Build history of the part. All positions in model axes, mm. Coordinates: 2 decimals unless noted, no trailing zeros. Loops run counter-clockwise (first coordinate to the right, second up) from the corner with the lowest first, then second, coordinate; pieces in that order, holes last.
Item 1: Cut at D-D (x = 8.5). List the corners of the cut face in (y, z).
Item 2: Cut at B-B (x = -11). List the corners of the cut face in (y, z), and give its area (3 significant figures).
Item 3: Drill centre lines: line 1 along Y through (x, z) = (-11, 1); line 2 along X through (y, z) = (-13, 1); line 3 along X through (y, z) = (-10, 1.25). Where is each one in solid material? Low to high.
Item 4: Cut at A-A (y = -13). List the corners of the cut face in (x, z).
Item 5: Cut at C-C (z = 2.3). List the corners of the cut face in (x, y), and give its area (3 significant figures).
Item 6: Mould opens along Y. For faces 1 (the face through (0, 0, 0)), 2 (the face through (-12.5, 13.07, 1.52)), 3 (the face through (0, -20, 1)), 4 (the face through (9.526, -11.352, 1.521)) say: released by +Y, released by -Y, zero draft, split by the parting line, or undercut.
from build123d import *

# Parameters (mm, degrees)
ESQUISSE1_W             = 28
ESQUISSE1_H             = 40
BOSS_EXTRU_1_DEPTH      = 3
ESQUISSE7_R             = 1.5
ENL_V_MAT_EXTRU_6_DEPTH = 5
ESQUISSE8_R             = 2
ENL_V_MAT_EXTRU_7_DEPTH = 10
ESQUISSE9_R             = 6
ENL_V_MAT_EXTRU_8_DEPTH = 10


with BuildPart() as part:
    # Esquisse1 → Boss.-Extru.1 (new body)
    with BuildSketch(Plane.XY):
        Rectangle(ESQUISSE1_W, ESQUISSE1_H)
    extrude(amount=BOSS_EXTRU_1_DEPTH)

    # Esquisse7 → Enlèv. mat.-Extru.6 (cut)
    with BuildSketch(Plane.XY.offset(3)):
        with Locations((-11, 13)):
            Circle(ESQUISSE7_R)
    enl_v_mat_extru_6 = extrude(amount=-ENL_V_MAT_EXTRU_6_DEPTH, mode=Mode.SUBTRACT)

    # Symétrie2: Enlèv. mat.-Extru.6 across plane
    add(enl_v_mat_extru_6.mirror(Plane.ZX), mode=Mode.SUBTRACT)

    # Esquisse8 → Enlèv. mat.-Extru.7 (cut)
    with BuildSketch(Plane.XY.offset(3)):
        with Locations((11, 10)):
            Circle(ESQUISSE8_R)
    enl_v_mat_extru_7 = extrude(amount=-ENL_V_MAT_EXTRU_7_DEPTH, mode=Mode.SUBTRACT)

    # Symétrie3: Enlèv. mat.-Extru.7 across plane
    add(enl_v_mat_extru_7.mirror(Plane.ZX), mode=Mode.SUBTRACT)

    # Esquisse9 → Enlèv. mat.-Extru.8 (cut)
    with BuildSketch(Plane.XY.offset(3)):
        with Locations((14, 0)):
            Circle(ESQUISSE9_R)
    extrude(amount=-ENL_V_MAT_EXTRU_8_DEPTH, mode=Mode.SUBTRACT)


solid = part.part
Filled sheet:
1. outline: (-20, 0) - (-2.4, 0) - (-2.4, 3) - (-20, 3) - close; (2.4, 0) - (20, 0) - (20, 3) - (2.4, 3) - close
2. outline: (-20, 0) - (-14.5, 0) - (-14.5, 3) - (-20, 3) - close; (-11.5, 0) - (11.5, 0) - (11.5, 3) - (-11.5, 3) - close; (14.5, 0) - (20, 0) - (20, 3) - (14.5, 3) - close
2. area: 102 mm2
3. line 1: y = -20 to -14.5, -11.5 to 11.5, 14.5 to 20
3. line 2: x = -14 to -12.5, -9.5 to 14
3. line 3: x = -14 to 9, 13 to 14
4. outline: (-14, 0) - (-12.5, 0) - (-12.5, 3) - (-14, 3) - close; (-9.5, 0) - (14, 0) - (14, 3) - (-9.5, 3) - close
5. outline: (-14, -20) - (14, -20) - (14, -6) arc R6 cw to (14, 6) - (14, 20) - (-14, 20) - close; hole circle Ø3 at (-11, -13); hole circle Ø3 at (-11, 13); hole circle Ø4 at (11, -10); hole circle Ø4 at (11, 10)
5. area: 1,020 mm2
6. face 1: zero draft
6. face 2: undercut
6. face 3: released by -Y
6. face 4: undercut
